Could you check a few things on this model? Use its own coordinates, in mm. Round coordinates to 2 decimals unless told otherwise and drop trailing zeros. Loops run counter-clockwise (first coordinate to the right, second up) from the corner with the lowest first, then second, coordinate; pieces in that order, holes last. Notation, with made-up numbers: M 20.5,7 L 39.5,7 A25 ccw 39.5,45 Z; hole C 56.5,74.5 d5. An arc over 180 degrees is marked long. Answer in a Markdown table with one row per item.
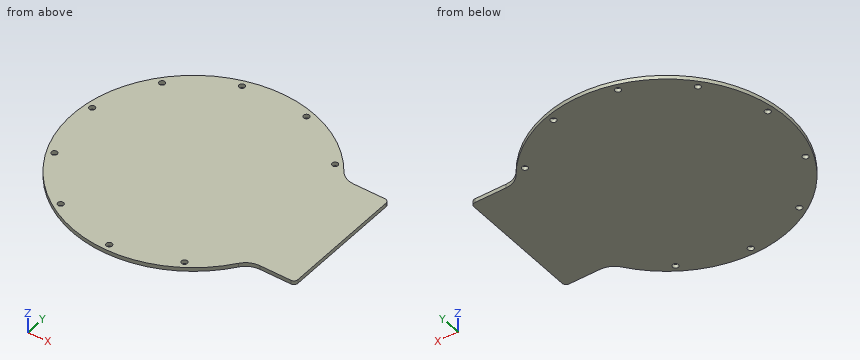
```python
from build123d import *

# Parameters (mm, degrees)
SKETCH_1_R      = 1.5
EXTRUDE_1_DEPTH = 2


with BuildPart() as part:
    # 草图1 → 凸台-拉伸1 (new body)
    with BuildSketch(Plane.XY):
        with BuildLine():
            Line((58.445187997, 32.9), (74.5685, 32.9))
            ThreePointArc((74.5685, 32.9), (75.982713562, 32.314213562), (76.5685, 30.9))
            Line((76.5685, 30.9), (76.5685, -30.9))
            ThreePointArc((76.5685, -30.9), (75.982713562, -32.314213562), (74.5685, -32.9))
            Line((74.5685, -32.9), (58.445187997, -32.9))
            ThreePointArc((58.445187997, -32.9), (53.927025417, -33.978889817), (50.383782756, -36.982758621))
            ThreePointArc((50.383782756, -36.982758621), (-62.5, 0), (50.383782756, 36.982758621))
            ThreePointArc((50.383782756, 36.982758621), (53.927025417, 33.978889817), (58.445187997, 32.9))
        make_face()
        with Locations((0, -59)):
            Circle(SKETCH_1_R, mode=Mode.SUBTRACT)
        with Locations((-31.89780823, -49.633958437)):
            Circle(SKETCH_1_R, mode=Mode.SUBTRACT)
        with Locations((-53.668287726, -24.509485767)):
            Circle(SKETCH_1_R, mode=Mode.SUBTRACT)
        with Locations((-58.399465071, 8.396575458)):
            Circle(SKETCH_1_R, mode=Mode.SUBTRACT)
        with Locations((-44.589224887, 38.636783303)):
            Circle(SKETCH_1_R, mode=Mode.SUBTRACT)
        with Locations((-16.622220854, 56.610085443)):
            Circle(SKETCH_1_R, mode=Mode.SUBTRACT)
        with Locations((16.622220854, 56.610085443)):
            Circle(SKETCH_1_R, mode=Mode.SUBTRACT)
        with Locations((44.589224887, 38.636783303)):
            Circle(SKETCH_1_R, mode=Mode.SUBTRACT)
        with Locations((31.89780823, -49.633958437)):
            Circle(SKETCH_1_R, mode=Mode.SUBTRACT)
    extrude(amount=EXTRUDE_1_DEPTH)


solid = part.part
```
1) I want a section at B-B, the plane y = -59. Please give me the cut outline in (x, z), plus the area to 3 significant figures.
Computed:
| item | result |
|---|---|
| outline | M -20.62,0 L -1.5,0 L -1.5,2 L -20.62,2 Z; M 1.5,0 L 20.62,0 L 20.62,2 L 1.5,2 Z |
| area | 76.5 mm² |
2) Will these pins go through, and if not, where does the flat tip stop? P1, Ø1, axis at y = 9, z = 1.5, coming from the -X side; P2, Ø4, axis at x = 31.9, y = -49.63, coming from the +Z side; P3, Ø1, axis at y = -11, z = 1, coming from the -X side; P4, Ø1, axis at x = 64.5, z = 1.5, coming from the -Y side.
Computed:
| item | result |
|---|---|
| P1 | stops at x = -61.92 |
| P2 | stops at z = 2 |
| P3 | stops at x = -61.61 |
| P4 | stops at y = -32.9 |
3) I want a section at D-D, the plane x = 53. Please give me the cut outline in (y, z), plus the area to 3 significant figures.
Computed:
| item | result |
|---|---|
| outline | M -34.51,0 L 34.51,0 L 34.51,2 L -34.51,2 Z |
| area | 138 mm² |
4) I need wall thicknesses on line 1 (Y direction, x = -53.5, z = 1.5); line 2 (X direction, y = 38, z = 1.4); line 3 (Y direction, x = 2, z = 1.95). Which ranges of each line are inside material? Lowest first, please.
Computed:
| item | result |
|---|---|
| line 1 | y = -32.31 to -26, -23.02 to 32.31 |
| line 2 | x = -49.62 to -45.95, -43.23 to 43.23, 45.95 to 49.62 |
| line 3 | y = -62.47 to 62.47 |
5) I want a section at A-A, the plane x = 0. Please give me the cut outline in (y, z).
Computed:
| item | result |
|---|---|
| outline | M -62.5,0 L -60.5,0 L -60.5,2 L -62.5,2 Z; M -57.5,0 L 62.5,0 L 62.5,2 L -57.5,2 Z |
6) I want a section at C-C, the plane z = 1.3. State how many separate pieces and enclosed holes the cut face has, plus the area to 3 significant figures.
Computed:
| item | result |
|---|---|
| separate pieces | 1 |
| enclosed holes | 9 |
| area | 13,300 mm² |
